```python
from build123d import *

# Parameters (mm, degrees)
SKETCH1_W             = 30
SKETCH1_H             = 34
BOSS_EXTRUDE1_DEPTH   = 22
F_4_0MM_DOWEL_HOLE1_D = 4
BOSS_EXTRUDE2_DEPTH   = 30
SKETCH5_W             = 30
SKETCH5_H             = 10.861011286
CUT_EXTRUDE1_DEPTH    = 1.5
CHAMFER2_SIZE         = 1.5
CUT_EXTRUDE2_DEPTH    = 41.902322672


with BuildPart() as part:
    # Sketch1 → Boss-Extrude1 (new body)
    with BuildSketch(Plane(origin=(0, 0, 0), x_dir=(1, 0, 0), z_dir=(0, 1, 0))):
        Rectangle(SKETCH1_W, SKETCH1_H)
    extrude(amount=BOSS_EXTRUDE1_DEPTH)

    # Ø4.0mm Dowel Hole1 (through all)
    with Locations(Plane(origin=(0, 22, 0), x_dir=(1, 0, 0), z_dir=(0, 1, 0))):
        with Locations((9, -12), (-9, -12), (9, 12), (-9, 12)):
            Hole(F_4_0MM_DOWEL_HOLE1_D / 2)

    # Sketch4 → Boss-Extrude2 (add, through all)
    with BuildSketch(Plane(origin=(15, 0, 0), x_dir=(0, 0, -1), z_dir=(1, 0, 0))):
        Polygon((-8.519809931, 0), (8.519809931, 0), (7.106209181, -2.5), (-7.106209181, -2.5), align=None)
    extrude(amount=-BOSS_EXTRUDE2_DEPTH)

    # Sketch5 → Cut-Extrude1 (cut)
    with BuildSketch(Plane(origin=(0, 22, 0), x_dir=(1, 0, 0), z_dir=(0, 1, 0))):
        Rectangle(SKETCH5_W, SKETCH5_H)
    extrude(amount=-CUT_EXTRUDE1_DEPTH, mode=Mode.SUBTRACT)

    # Chamfer2
    chamfer2_edges = [part.edges().sort_by_distance(p)[0] for p in [
        (0, 20.5, 5.430505643),
        (0, 20.5, -5.430505643),
    ]]
    chamfer(chamfer2_edges, length=CHAMFER2_SIZE - 0.0001)  # a hair under: the kernel refuses the full size

    # Sketch8 → Cut-Extrude2 (cut, through all)
    with BuildSketch(Plane(origin=(15, 0, 0), x_dir=(0, 0, -1), z_dir=(1, 0, 0))):
        with BuildLine():
            Line((4, 11), (0, 11))
            Line((0, 11), (-4, 11))
            ThreePointArc((-4, 11), (0, 7), (4, 11))
        make_face()
        with BuildLine():
            Line((-4, 11), (0, 11))
            Line((0, 11), (4, 11))
            ThreePointArc((4, 11), (0, 15), (-4, 11))
        make_face()
    extrude(amount=-CUT_EXTRUDE2_DEPTH, mode=Mode.SUBTRACT)


solid = part.part
```
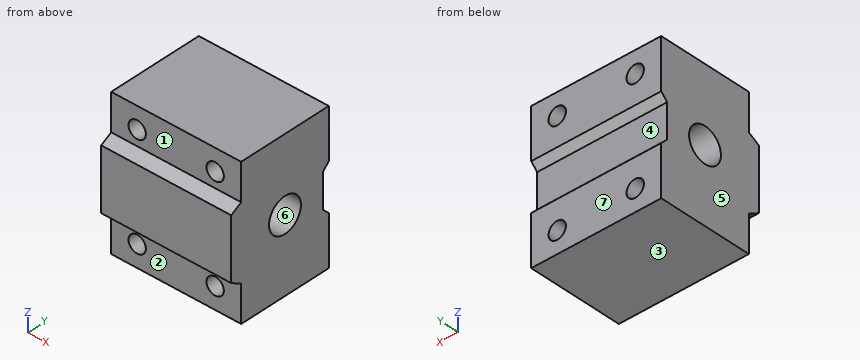
Source: CAD feature listing. Evaluate the final solid. Frame: model axes, mm. Face numbers are marked on the shaded views. A direction names the side the tool comes from. Give positions to 0.01 mm unless a question says otherwise; leave off trailing zeros. Loops run counter-clockwise (first coordinate to the right, second up) from the corner with the lowest first, then second, coordinate; pieces in that order, holes last. Notation, with made-up numbers: (5, 78.5) -> (45, 78.5) arc R8 cw to (45, 84.5) -> close; hole circle Ø6 at (-33.5, -5). An arc over 180 degrees is marked (long way). Put each result on its own line as item: value. Start each with the question number.
1) Reachability of the marked faces 1, 2, 3 and 4 from +Z, -Z, +X, -X, +Y, -Y: full face, straight path, thin tool, end or side. Return the list, or none.
2) Material intervals for probe 1 along Y at (x, z) = (-2.5, 0); probe 2 along Z at (x, y) = (-9, 17); probe 3 along Z at (x, y) = (-8.5, 8.75), sorted ascending.
3) Draft query along Y for the marked faces 5, 6 and 7. Return one class per face: released by +Y, released by -Y, zero draft, split by the parting line, or undercut.
4) Cut plane D-D (y = 1.75). Return loops of the section in (x, z).
5) Cut plane C-C (z = -12). Return loops of the section in (x, y).
6) Cut plane A-A (x = 9). State how many separate pieces and enclosed holes the cut face has, then the cut area to 3 significant figures.
7) Contact query for flat-ended pins moving along their axis: P1, Ø2.5, axis at x = 9, z = 12, coming from the -Y side; P2, Ø7, axis at x = 5.5, z = -13, coming from the -Y side; P3, Ø4, axis at x = 3.5, z = 0, coming from the +Y side. Output: stop coordinate, or through.
8) Cut plane B-B (z = 0). Return loops of the section in (x, y).
Results are:
1. face 1: +Z, +X, -X, -Y
1. face 2: -Z, +X, -X, -Y
1. face 3: -Z, +X, -X, +Y, -Y
1. face 4: +X, -X, +Y
2. probe 1: y = -2.5 to 7, 15 to 20.5
2. probe 2: z = -17 to -14, -10 to 10, 14 to 17
2. probe 3: z = -17 to -13.94, -10.06 to -3.31, 3.31 to 10.06, 13.94 to 17
3. face 5: zero draft
3. face 6: undercut
3. face 7: released by +Y
4. outline: (-15, -17) -> (15, -17) -> (15, 17) -> (-15, 17) -> close; hole circle Ø4 at (-9, -12); hole circle Ø4 at (-9, 12); hole circle Ø4 at (9, -12); hole circle Ø4 at (9, 12)
5. outline: (-15, 0) -> (-11, 0) -> (-11, 22) -> (-15, 22) -> close; (-7, 0) -> (7, 0) -> (7, 22) -> (-7, 22) -> close; (11, 0) -> (15, 0) -> (15, 22) -> (11, 22) -> close
6. separate pieces: 3
6. enclosed holes: 1
6. area: 547 mm2
7. P1: passes through
7. P2: stops at y = 0
7. P3: stops at y = 20.5
8. outline: (-15, -2.5) -> (15, -2.5) -> (15, 7) -> (-15, 7) -> close; (-15, 15) -> (15, 15) -> (15, 20.5) -> (-15, 20.5) -> close
